Source: CAD feature listing. Evaluate the final solid. Frame: model axes, mm. Round coordinates to 2 decimals unless told otherwise and drop trailing zeros. Order: outer loops, then holes, each group sorted by start corner. A loop starts at its lowest first (then second) coordinate and runs counter-clockwise, first axis right, second up. Notation, with made-up numbers: (85, -16.75) -> (142, -16.75) arc R10 ccw to (142, -11.75) -> close; hole circle Ø5 at (-26, 44.5). An arc over 180 degrees is marked (long way). Write item = value, one per line. Start each with the question number.
(1) Cut plane A-A on z = 0. Return the cut outline in (x, y), then the cut area to 3 significant figures.
(2) Draft query along Z for faces 1 (the face through (-48.33, 6, 0.19)), 2 (the face through (-3.034, 7.716, 68.933)), 3 (the face through (30, 0, 1)). Return one class per face: released by +Z, released by -Z, zero draft, split by the parting line, or undercut.
(3) Ray query, line 1 (Z direction, x = -37.5, y = 3); line 2 (X direction, y = 3.5, z = -47.5); line 3 (Y direction, x = -54, z = 1.5). Return the intervals inside material, ascending.
(4) Contact query for flat-ended pins moving along their axis: pin 1 Ø4 at (x, y) = (24, 7) entering from +Z; pin 2 Ø8 at (x, y) = (50, 7.5) entering from +Z; pin 3 Ø3 at (x, y) = (40, 2.5) entering from -Z. Output: stop coordinate, or through.
(5) Cut plane B-B on x = 0. Return the cut outline in (y, z).
from build123d import *

# Parameters (mm, degrees)
TAGLIO_ESTRUSIONE5_START    = -2
SCHIZZO2_R                  = 12.5
TAGLIO_ESTRUSIONE5_DEPTH    = 12
RIPETIZIONECIRCOLARE1_COUNT = 3


with BuildPart() as part:
    # Schizzo1 → Rivoluzione1 (revolve)
    with BuildSketch(Plane.XY, mode=Mode.PRIVATE) as rivoluzione1_sk:
        Polygon((-69, 15.650720073), (-69, 0), (-26, 0), align=None)
    revolve(rivoluzione1_sk.sketch.rotate(Axis((0, 0, 0), (0, 1, 0)), 270), axis=Axis((0, 0, 0), (0, 1, 0)))

    # Schizzo2 → Taglio-Estrusione5 (cut)
    with BuildSketch(Plane(origin=(-3.041422239, -8.356238926, 6.34e-07), x_dir=(-0.9396926207859105, 0.3420201433256629, 0), z_dir=(0.34202014332566205, 0.9396926207859082, -7.133604585251575e-08)).offset(TAGLIO_ESTRUSIONE5_START)):
        with Locations(Location((47.311830249, -6.33e-07, 0), (0, 0, 276.586310477))):
            Circle(SCHIZZO2_R)
    taglio_estrusione5 = extrude(amount=TAGLIO_ESTRUSIONE5_DEPTH, mode=Mode.SUBTRACT)

    # RipetizioneCircolare1: Taglio-Estrusione5 ×3 about axis
    ripetizionecircolare1_axis = Axis((0, 0, 0), (0, 1, 0))
    for i in range(1, RIPETIZIONECIRCOLARE1_COUNT):
        add(taglio_estrusione5.rotate(ripetizionecircolare1_axis, i * 360 / RIPETIZIONECIRCOLARE1_COUNT), mode=Mode.SUBTRACT)


solid = part.part
Evaluation:
q1.outline = (-69, 0) -> (-26, 0) -> (-35.75, 3.55) -> (-36.44, 1.67) -> (-59.93, 10.22) -> (-59.25, 12.1) -> (-69, 15.65) -> close; (26, 0) -> (69, 0) -> (69, 15.65) -> close
q1.area = 623 mm^2
q2.face_1 = undercut
q2.face_2 = split by the parting line
q2.face_3 = zero draft
q3.line_1 = -57.92 to -5.85, 5.85 to 57.92
q3.line_2 = -50.05 to 50.05
q3.line_3 = 0 to 8.06
q4.pin_1 = 65.4
q4.pin_2 = 51.43
q4.pin_3 = -57.26
q5.outline = (0, -69) -> (15.65, -69) -> (0, -26) -> close; (0, 26) -> (15.65, 69) -> (0, 69) -> close
